Read the model definition and answer for the solid it produces. Units are mm, in the model's axes. A direction names the side the tool comes from. Coordinates: 2 decimals unless noted, no trailing zeros. Loops run counter-clockwise (first coordinate to the right, second up) from the corner with the lowest first, then second, coordinate; pieces in that order, holes last. Notation, with made-up numbers: M 24,73.5 L 73,73.5 A29 ccw 73,111.5 Z; hole C 82,51.25 d11. An arc over 180 degrees is marked long. Use one line per item in the form item = value. Start each with the question number.
1. Find the intervals of material crossed by probe 1 along Z at (x, y) = (158.5, 1.85); probe 2 along Z at (x, y) = (101, 2.75); probe 3 along X at (y, z) = (2.05, -125), in increasing order. Write a range as [from, to].
2. The part is cut by section B-B (z = -24). Give the vertices of the cut face in (x, y).
3. A tool of negligible diameter and unlimited length cuts with its end or side. For faces 3 (the flat face through (107, 0, -182)), 4 (the cylindrical face through (10.57, 2.03, -11.36)), from which of +Z, -Z, +X, -X, +Y, -Y can it reach the whole face along a straight path? Write none if from no direction.
4. The part is cut by section C-C (y = 3.3). Give the number of separate pieces and of enclosed holes in the cut face, plus the area to 3 significant figures.
5. For a pull along X with two mould halves and no side action, classify faces 1 (the flat face through (107, 4, -182)), 2 (the cylindrical face through (11, 2, -188)) as released by +X, released by -X, zero draft, split by the parting line, or undercut.
6. The part is cut by section A-A (x = 34.5). Give the vertices of the cut face in (y, z), plus the area to 3 significant figures.
from build123d import *

# Parameters (mm, degrees)
CROQUIS1_W              = 200
CROQUIS1_H              = 200
CROQUIS1_R              = 2.5
SALIENTE_EXTRUIR1_DEPTH = 4
CROQUIS2_W              = 158
CROQUIS2_H              = 158
CORTAR_EXTRUIR1_DEPTH   = 10
CROQUIS4_W              = 4
CROQUIS4_H              = 15
CROQUIS4_W_2            = 15
CROQUIS4_H_2            = 4
CORTAR_EXTRUIR2_DEPTH   = 10


with BuildPart() as part:
    # Croquis1 → Saliente-Extruir1 (new body)
    with BuildSketch(Plane(origin=(0, 0, 0), x_dir=(1, 0, 0), z_dir=(0, 1, 0))):
        with Locations((100, 100)):
            Rectangle(CROQUIS1_W, CROQUIS1_H)
        with Locations(Location((15, 185, 0), (0, 0, 270))):
            Circle(CROQUIS1_R, mode=Mode.SUBTRACT)
        with Locations(Location((185, 185, 0), (0, 0, 270))):
            Circle(CROQUIS1_R, mode=Mode.SUBTRACT)
        with Locations(Location((185, 15, 0), (0, 0, 270))):
            Circle(CROQUIS1_R, mode=Mode.SUBTRACT)
        with Locations(Location((15, 15, 0), (0, 0, 270))):
            Circle(CROQUIS1_R, mode=Mode.SUBTRACT)
    extrude(amount=SALIENTE_EXTRUIR1_DEPTH)

    # Croquis2 → Cortar-Extruir1 (cut)
    with BuildSketch(Plane(origin=(0, 4, 0), x_dir=(1, 0, 0), z_dir=(0, 1, 0))):
        with Locations((100, 100)):
            Rectangle(CROQUIS2_W, CROQUIS2_H)
    extrude(amount=-CORTAR_EXTRUIR1_DEPTH, mode=Mode.SUBTRACT)

    # Croquis4 → Cortar-Extruir2 (cut)
    with BuildSketch(Plane(origin=(0, 4, 0), x_dir=(1, 0, 0), z_dir=(0, 1, 0))):
        with Locations((10.5, 130.833333333)):
            Rectangle(CROQUIS4_W, CROQUIS4_H)
        with Locations((10.5, 161.666666667)):
            Rectangle(CROQUIS4_W, CROQUIS4_H)
        with Locations((38.333333333, 189.5)):
            Rectangle(CROQUIS4_W_2, CROQUIS4_H_2)
        with Locations((72.916666667, 189.5)):
            Rectangle(CROQUIS4_W_2, CROQUIS4_H_2)
        with Locations((189.564602861, 126.146591855)):
            Rectangle(CROQUIS4_W, CROQUIS4_H)
        with Locations((189.564602861, 160.729925188)):
            Rectangle(CROQUIS4_W, CROQUIS4_H)
        with Locations((130.897936194, 188.563258522)):
            Rectangle(CROQUIS4_W_2, CROQUIS4_H_2)
        with Locations((161.731269527, 188.563258522)):
            Rectangle(CROQUIS4_W_2, CROQUIS4_H_2)
        with Locations((126.211194716, 9.498655661)):
            Rectangle(CROQUIS4_W_2, CROQUIS4_H_2)
        with Locations((160.794528049, 9.498655661)):
            Rectangle(CROQUIS4_W_2, CROQUIS4_H_2)
        with Locations((188.627861382, 68.165322328)):
            Rectangle(CROQUIS4_W, CROQUIS4_H)
        with Locations((188.627861382, 37.331988994)):
            Rectangle(CROQUIS4_W, CROQUIS4_H)
        with Locations((9.563258522, 72.852063806)):
            Rectangle(CROQUIS4_W, CROQUIS4_H)
        with Locations((9.563258522, 38.268730473)):
            Rectangle(CROQUIS4_W, CROQUIS4_H)
        with Locations((68.229925188, 10.435397139)):
            Rectangle(CROQUIS4_W_2, CROQUIS4_H_2)
        with Locations((37.396591855, 10.435397139)):
            Rectangle(CROQUIS4_W_2, CROQUIS4_H_2)
        with Locations((100, 189.5)):
            Rectangle(CROQUIS4_W_2, CROQUIS4_H_2)
        with Locations((10.5, 100)):
            Rectangle(CROQUIS4_W, CROQUIS4_H)
        with Locations((189.5, 100)):
            Rectangle(CROQUIS4_W, CROQUIS4_H)
        with Locations((100, 10.5)):
            Rectangle(CROQUIS4_W_2, CROQUIS4_H_2)
        with BuildLine():
            ThreePointArc((15, 192.5), (9.696699141, 190.303300859), (7.5, 185))
            ThreePointArc((7.5, 185), (8.75, 183.75), (10, 185))
            ThreePointArc((10, 185), (11.464466094, 188.535533906), (15, 190))
            ThreePointArc((15, 190), (16.25, 191.25), (15, 192.5))
        make_face()
        with BuildLine():
            ThreePointArc((185.064602861, 191.563258522), (183.814602861, 190.313258522), (185.064602861, 189.063258522))
            ThreePointArc((185.064602861, 189.063258522), (188.600136767, 187.598792428), (190.064602861, 184.063258522))
            ThreePointArc((190.064602861, 184.063258522), (191.314602861, 182.813258522), (192.564602861, 184.063258522))
            ThreePointArc((192.564602861, 184.063258522), (190.367903719, 189.366559381), (185.064602861, 191.563258522))
        make_face()
        with BuildLine():
            ThreePointArc((191.627861382, 13.998655661), (190.377861382, 15.248655661), (189.127861382, 13.998655661))
            ThreePointArc((189.127861382, 13.998655661), (187.663395288, 10.463121755), (184.127861382, 8.998655661))
            ThreePointArc((184.127861382, 8.998655661), (182.877861382, 7.748655661), (184.127861382, 6.498655661))
            ThreePointArc((184.127861382, 6.498655661), (189.431162241, 8.695354802), (191.627861382, 13.998655661))
        make_face()
        with BuildLine():
            ThreePointArc((14.063258522, 7.435397139), (15.313258522, 8.685397139), (14.063258522, 9.935397139))
            ThreePointArc((14.063258522, 9.935397139), (10.527724616, 11.399863233), (9.063258522, 14.935397139))
            ThreePointArc((9.063258522, 14.935397139), (7.813258522, 16.185397139), (6.563258522, 14.935397139))
            ThreePointArc((6.563258522, 14.935397139), (8.759957663, 9.632096281), (14.063258522, 7.435397139))
        make_face()
    extrude(amount=-CORTAR_EXTRUIR2_DEPTH, mode=Mode.SUBTRACT)


solid = part.part
Computed values:
q1.probe_1 = [-200, -190.56], [-186.56, -179], [-21, -11.5], [-7.5, 0]
q1.probe_2 = [-200, -191.5], [-187.5, -179], [-21, -12.5], [-8.5, 0]
q1.probe_3 = [0, 8.5], [12.5, 21], [179, 187.56], [191.56, 200]
q2.outline = M 0,0 L 21,0 L 21,4 L 0,4 Z; M 179,0 L 200,0 L 200,4 L 179,4 Z
q3.face_3 = +Z, -Z, +X, -X, -Y
q3.face_4 = +Y, -Y
q4.separate_pieces = 1
q4.enclosed_holes = 29
q4.area = 13,600 mm²
q5.face_1 = zero draft
q5.face_2 = undercut
q6.outline = M 0,-200 L 4,-200 L 4,-191.5 L 0,-191.5 Z; M 0,-187.5 L 4,-187.5 L 4,-179 L 0,-179 Z; M 0,-21 L 4,-21 L 4,-12.44 L 0,-12.44 Z; M 0,-8.44 L 4,-8.44 L 4,0 L 0,0 Z
q6.area = 136 mm²
